Build history of the part. All positions in model axes, mm. Coordinates: 2 decimals unless noted, no trailing zeros. Write each loop counter-clockwise with the first axis right and the second up, starting at its lowest first coordinate (ties: lowest second). Pieces come first, ordered by that corner, then holes. Notation, with made-up numbers: (62.25, -22) -> (80.25, -22) arc R16 cw to (80.25, -2) -> close; hole circle Ø8 at (77.25, 24). An arc over 180 degrees is marked (long way). Write each question's results on one line, items separated by ' | '. Start each with the question number.
Q1. Drill centre lines: line 1 (Y direction, x = 41.75, z = 31); line 2 (Y direction, x = 37.5, z = -14). Where is each one in solid material? Low to high.
Q2. Drop flat-ended pins along their axis: pin 1 Ø1 at (x, z) = (44, 28.5) entering from +Y; pin 2 Ø1 at (x, z) = (40, -31) entering from +Y. Give the stop position or say it passes through.
Q3. Saw through at A-A on x = 42.5. Give the cut face in (y, z), and give its area (3 significant figures).
Q4. Saw through at B-B on z = -22. Give the cut face in (x, y), and give its area (3 significant figures).
from build123d import *

# Parameters (mm, degrees)
F0_W     = 11.43
F0_H     = 109.728
F1_DEPTH = 7.62
F3_DEPTH = 25.4


with BuildPart() as f1:
    # F0 (on Front) → F1 (new body)
    with BuildSketch(Plane.XZ):
        with Locations((41.4564540316, 10.5215980716)):
            Rectangle(F0_W, F0_H)
    extrude(amount=F1_DEPTH)

    # F2 (on face) → F3 (cut)
    with BuildSketch(Plane.YZ.offset(47.1714540316)):
        with BuildLine():
            ThreePointArc((0, 32.3497010216), (-1.2394704753, -6.0294134076), (-3.81, -44.3424019284))
            Line((-3.81, -44.3424019284), (0, -44.3424019284))
            Line((0, -44.3424019284), (0, 32.3497010216))
        make_face()
    extrude(amount=-F3_DEPTH, mode=Mode.SUBTRACT)


solid = f1.part
Returned:
1) line 1: y = -7.62 to -0.02 | line 2: y = -7.62 to -1.66
2) pin 1: stops at y = -0.06 | pin 2: stops at y = -2.73
3) outline: (-7.62, -44.34) -> (-3.81, -44.34) arc R1106.39 ccw to (0, 32.35) -> (0, 65.39) -> (-7.62, 65.39) -> close | area: 724 mm2
4) outline: (35.74, -7.62) -> (47.17, -7.62) -> (47.17, -2.15) -> (35.74, -2.15) -> close | area: 62.5 mm2
